```python
from build123d import *

# Parameters (mm, degrees)
SKETCH1_R           = 15
SKETCH1_R_2         = 2.375
SKETCH1_R_3         = 2.9
SKETCH1_R_4         = 10.65
BOSS_EXTRUDE1_DEPTH = 8


with BuildPart() as part:
    # Sketch1 → Boss-Extrude1 (new body)
    with BuildSketch(Plane(origin=(0, 0, 0), x_dir=(1, 0, 0), z_dir=(0, 1, 0))):
        Polygon((8, 191.154701829), (8, 190), (0, 190), (0, 0), (420, 0), (420, 190), (412, 190), (412, 191.154701829), align=None)
        with Locations(Location((300, 137, 0), (0, 0, 270))):
            Circle(SKETCH1_R, mode=Mode.SUBTRACT)
        with Locations(Location((300, 53, 0), (0, 0, 270))):
            Circle(SKETCH1_R, mode=Mode.SUBTRACT)
        with Locations(Location((258, 95, 0), (0, 0, 270))):
            Circle(SKETCH1_R, mode=Mode.SUBTRACT)
        with Locations(Location((300, 95, 0), (0, 0, 270))):
            Circle(SKETCH1_R, mode=Mode.SUBTRACT)
        with Locations(Location((342, 95, 0), (0, 0, 270))):
            Circle(SKETCH1_R, mode=Mode.SUBTRACT)
        with BuildLine():
            Line((112.209434277, 135.177360592), (112.209434277, 137.577360592))
            ThreePointArc((112.209434277, 137.577360592), (114.809434277, 140.177360592), (117.409434277, 137.577360592))
            Line((117.409434277, 137.577360592), (117.409434277, 135.177360592))
            ThreePointArc((117.409434277, 135.177360592), (114.809434277, 132.577360592), (112.209434277, 135.177360592))
        make_face(mode=Mode.SUBTRACT)
        with Locations(Location((104.809434277, 136.82735285, 0), (0, 0, 270))):
            Circle(SKETCH1_R_2, mode=Mode.SUBTRACT)
        with BuildLine():
            Line((72.209434277, 53.577360592), (72.209434277, 55.977360592))
            ThreePointArc((72.209434277, 55.977360592), (74.809434277, 58.577360592), (77.409434277, 55.977360592))
            Line((77.409434277, 55.977360592), (77.409434277, 53.577360592))
            ThreePointArc((77.409434277, 53.577360592), (74.809434277, 50.977360592), (72.209434277, 53.577360592))
        make_face(mode=Mode.SUBTRACT)
        with Locations(Location((84.809434277, 54.327360592, 0), (0, 0, 270))):
            Circle(SKETCH1_R_2, mode=Mode.SUBTRACT)
        with Locations(Location((94.809434277, 54.327360592, 0), (0, 0, 270))):
            Circle(SKETCH1_R_3, mode=Mode.SUBTRACT)
        with BuildLine():
            Line((112.209434277, 53.577360592), (112.209434277, 55.977360592))
            ThreePointArc((112.209434277, 55.977360592), (114.809434277, 58.577360592), (117.409434277, 55.977360592))
            Line((117.409434277, 55.977360592), (117.409434277, 53.577360592))
            ThreePointArc((117.409434277, 53.577360592), (114.809434277, 50.977360592), (112.209434277, 53.577360592))
        make_face(mode=Mode.SUBTRACT)
        with Locations(Location((94.809434277, 95.577360592, 0), (0, 0, 270))):
            Circle(SKETCH1_R_4, mode=Mode.SUBTRACT)
        with BuildLine():
            Line((77.409434277, 137.577360592), (77.409434277, 135.177360592))
            ThreePointArc((77.409434277, 135.177360592), (74.809434277, 132.577360592), (72.209434277, 135.177360592))
            Line((72.209434277, 135.177360592), (72.209434277, 137.577360592))
            ThreePointArc((72.209434277, 137.577360592), (74.809434277, 140.177360592), (77.409434277, 137.577360592))
        make_face(mode=Mode.SUBTRACT)
        with Locations(Location((94.809434277, 136.827360592, 0), (0, 0, 270))):
            Circle(SKETCH1_R_3, mode=Mode.SUBTRACT)
    extrude(amount=BOSS_EXTRUDE1_DEPTH)


solid = part.part
```
Here's how the part is built. I have some questions about the finished solid (model axes, mm). A direction names the side the tool comes from. Coordinates: 2 decimals unless noted, no trailing zeros. Order: outer loops, then holes, each group sorted by start corner. A loop starts at its lowest first (then second) coordinate and runs counter-clockwise, first axis right, second up.
1) Which directions (+Z, -Z, +X, -X, +Y, -Y) give clear straight access to the entire face, cutting with the end or side of a thin tool? Please do faces 5 (the face through (4, 4, -190)), 6 (the face through (314.872, 3.944, -96.953)), 7 (the face through (416, 4, -190)).
2) Imagine slicing it at D-D on y = 2.5. State how many separate pieces and enclosed holes the cut face has, and give its area (3 significant figures).
3) Imagine slicing it at A-A on x = 258. List the corners of the cut face in (y, z) for me.
4) I need wall thicknesses on line 1 (X direction, y = 3.25, z = -95); line 2 (X direction, y = 4.75, z = -137); line 3 (Z direction, x = 301, y = 4.5). Which ranges of each line are inside material? Lowest first, please.
5) Imagine slicing it at B-B on x = 300. List the corners of the cut face in (y, z) for me.
6) Will these pins go through, and if not, where does the flat tip stop? pin 1 (19 mm diameter, centred on x = 94.81, z = -95.58, fed in from +Y); pin 2 (1.2 mm diameter, centred on y = 5, z = -55, fed in from -X); pin 3 (0.6 mm diameter, centred on y = 4, z = -190.5, fed in from -X).
7) Imagine slicing it at C-C on z = -95. List the corners of the cut face in (x, y) for me.
8) We'd pull the mould along Z, two halves only. Please class faces 1 (the face through (213, 4, -191.155)), 2 (the face through (314.872, 3.944, -138.953)), 3 (the face through (0, 4, -96)), 4 (the face through (356.872, 3.944, -96.953)): +Z half, -Z half, draft (parallel to the pull), parting line (faces both ways), or undercut.
Response values:
1. face 5: -Z, -X, +Y, -Y
1. face 6: +Y, -Y
1. face 7: -Z, +X, +Y, -Y
2. separate pieces: 1
2. enclosed holes: 14
2. area: 76,200 mm2
3. outline: (0, -191.15) - (8, -191.15) - (8, -110) - (0, -110) - close; (0, -80) - (8, -80) - (8, 0) - (0, 0) - close
4. line 1: x = 0 to 84.18, 105.44 to 243, 273 to 285, 315 to 327, 357 to 420
4. line 2: x = 0 to 72.21, 77.41 to 91.91, 97.7 to 102.44, 107.18 to 112.21, 117.41 to 285, 315 to 420
4. line 3: z = -191.15 to -151.97, -122.03 to -109.97, -80.03 to -67.97, -38.03 to 0
5. outline: (0, -191.15) - (8, -191.15) - (8, -152) - (0, -152) - close; (0, -122) - (8, -122) - (8, -110) - (0, -110) - close; (0, -80) - (8, -80) - (8, -68) - (0, -68) - close; (0, -38) - (8, -38) - (8, 0) - (0, 0) - close
6. pin 1: passes through
6. pin 2: stops at x = 0
6. pin 3: stops at x = 8
7. outline: (0, 0) - (84.18, 0) - (84.18, 8) - (0, 8) - close; (105.44, 0) - (243, 0) - (243, 8) - (105.44, 8) - close; (273, 0) - (285, 0) - (285, 8) - (273, 8) - close; (315, 0) - (327, 0) - (327, 8) - (315, 8) - close; (357, 0) - (420, 0) - (420, 8) - (357, 8) - close
8. face 1: -Z half
8. face 2: undercut
8. face 3: draft
8. face 4: undercut
